Job drawing, mm, ordinate dimensions from the low corner. One solid piece. A direction names the side the tool comes from. Give positions to 0.01 mm unless a question says otherwise; leave off trailing zeros. Order: outer loops, then holes, each group sorted by start corner. A loop starts at its lowest first (then second) coordinate and runs counter-clockwise, first axis right, second up. Notation, with made-up numbers: M 86.25,-32 L 129.25,-32 A19 cw 129.25,2 Z; hole C -3.5,-26 d8. An arc over 180 degrees is marked long. One line per question, with ' | ' between items.
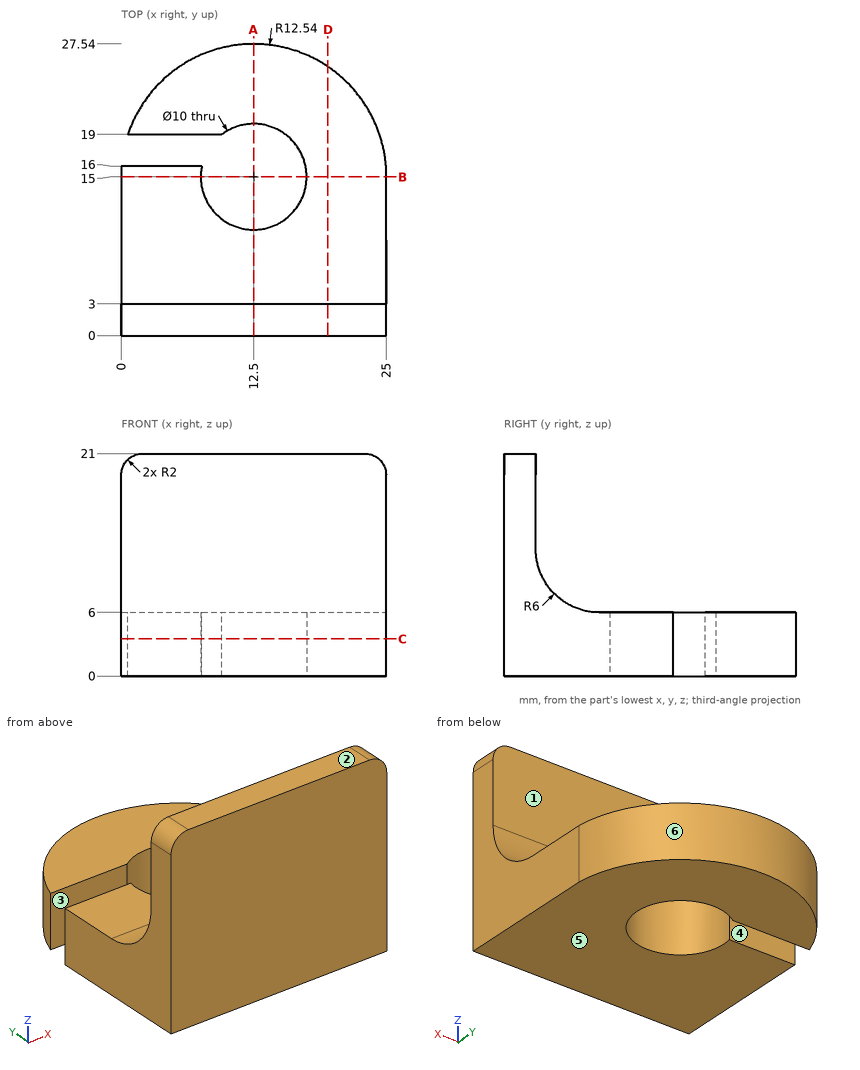
1. Slice it at C-C on z = 3.5. Give the cut face in (x, y) (3 decimals).
Worked out:
outline: M 0,0 L 25,0 L 25,16 A12.54 ccw 0.615,19 L 9.5,19 A5 cw long 7.601,16 L 0,16 Z
2. Tool access for the marked faces 1, 2 and 3: list every direction of +Z, -Z, +X, -X, +Y, -Y with a clear straight run to the whole face (end or side of a thin tool).
Worked out:
face 1: +Z, +X, -X, +Y | face 2: +Z, +X, -X, +Y, -Y | face 3: +Z, -Z, -X
3. Mould opens along Y. For the marked faces 4, 5 and 6 say: released by +Y, released by -Y, zero draft, split by the parting line, or undercut.
Worked out:
face 4: undercut | face 5: zero draft | face 6: released by +Y
4. Slice it at A-A on x = 12.5. Give the cut face in (y, z).
Worked out:
outline: M 0,0 L 10,0 L 10,6 L 9,6 A6 cw 3,12 L 3,21 L 0,21 Z; M 20,0 L 27.54,0 L 27.54,6 L 20,6 Z
5. Slice it at D-D on x = 19.5. Give the cut face in (y, z).
Worked out:
outline: M 0,0 L 25.4,0 L 25.4,6 L 9,6 A6 cw 3,12 L 3,21 L 0,21 Z
6. Probe L1, parallel to X at y = 15, z = 3.1; L2, parallel to Z at x = 6.5, y = 21; L3, parallel to Y at x = 3.5, z = 18.5. List the from-to ranges inside material, lowest first. Write a range as from..to.
Worked out:
L1: x = 0..7.5, 17.5..25 | L2: z = 0..6 | L3: y = 0..3
7. Drop flat-ended pins along their axis: pin 1 (7 mm diameter, centred on x = 16.5, z = 16, fed in from +Y); pin 2 (3 mm diameter, centred on x = 16.5, y = 6, fed in from +Z); pin 3 (3 mm diameter, centred on x = 5.5, z = 4, fed in from +Y). Give the stop position or say it passes through.
Worked out:
pin 1: stops at y = 3 | pin 2: stops at z = 8.03 | pin 3: stops at y = 26.27
8. Slice it at B-B on y = 15. Give the cut face in (x, z).
Worked out:
outline: M 0,0 L 7.5,0 L 7.5,6 L 0,6 Z; M 17.5,0 L 25,0 L 25,6 L 17.5,6 Z
